Could you check a few things on this drawing? It's one solid part, dimensions in mm from its lowest x, y, z. Round coordinates to 2 decimals unless told otherwise and drop trailing zeros. Loops run counter-clockwise (first coordinate to the right, second up) from the corner with the lowest first, then second, coordinate; pieces in that order, holes last. Notation, with made-up numbers: M 76,9.5 L 95,9.5 A17 cw 95,23.5 Z; hole C 14.5,-3.75 d11. An arc over 180 degrees is marked long. Answer as a JSON object with one key per item and string values.
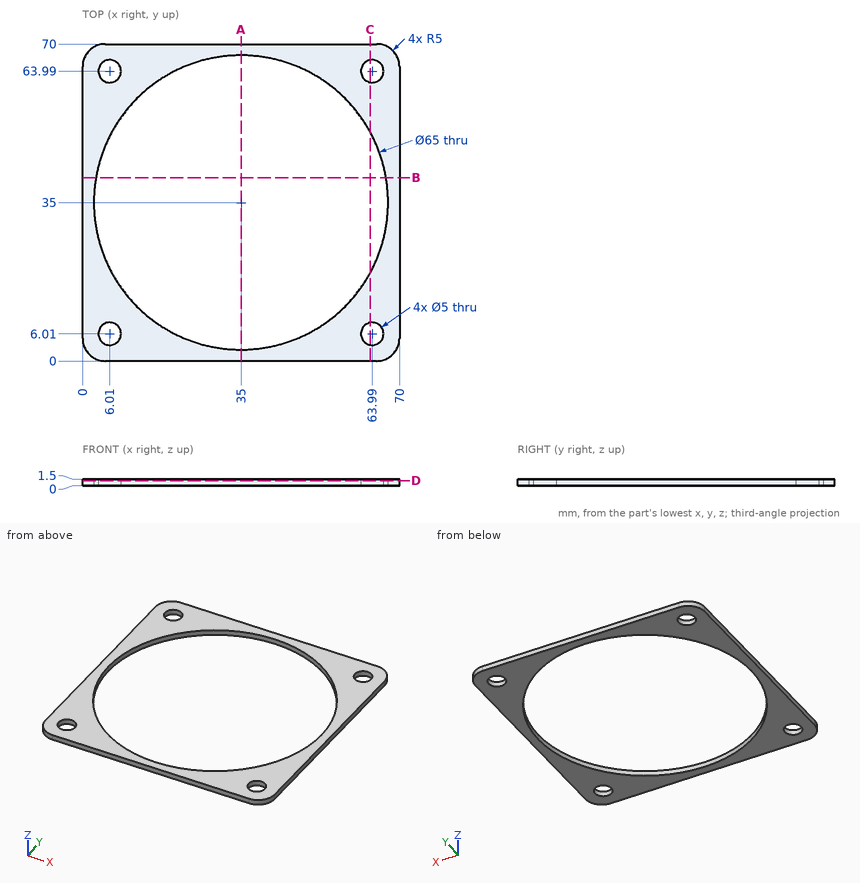
Item 1: I want a section at A-A, the plane x = 35. Please give me the cut outline in (y, z).
Resolved:
{"outline": "M 0,0 L 2.5,0 L 2.5,1.5 L 0,1.5 Z; M 67.5,0 L 70,0 L 70,1.5 L 67.5,1.5 Z"}
Item 2: I want a section at C-C, the plane x = 63.5. Please give me the cut outline in (y, z).
Resolved:
{"outline": "M 0,0 L 3.56,0 L 3.56,1.5 L 0,1.5 Z; M 8.46,0 L 19.38,0 L 19.38,1.5 L 8.46,1.5 Z; M 50.62,0 L 61.54,0 L 61.54,1.5 L 50.62,1.5 Z; M 66.44,0 L 70,0 L 70,1.5 L 66.44,1.5 Z"}
Item 3: I want a section at B-B, the plane y = 40.5. Please give me the cut outline in (x, z).
Resolved:
{"outline": "M 0,0 L 2.97,0 L 2.97,1.5 L 0,1.5 Z; M 67.03,0 L 70,0 L 70,1.5 L 67.03,1.5 Z"}
Item 4: I want a section at D-D, the plane z = 1.15. Please give me the cut outline in (x, y).
Resolved:
{"outline": "M 0,5 A5 ccw 5,0 L 65,0 A5 ccw 70,5 L 70,65 A5 ccw 65,70 L 5,70 A5 ccw 0,65 Z; hole C 35,35 d65; hole C 6.01,6.01 d5; hole C 6.01,63.99 d5; hole C 63.99,6.01 d5; hole C 63.99,63.99 d5"}
Item 5: Please list where these lines run through material, in increasing order: probe 1 along Y at (x, z) = (64, 0.3) (1 decimal); probe 2 along Y at (x, z) = (5, 1.25) (1 decimal); probe 3 along X at (y, z) = (29.5, 0.5). Write a range as from..to.
Resolved:
{"probe 1": "0..3.5, 8.5..20.3, 49.7..61.5, 66.5..70", "probe 2": "0..3.7, 8.3..22.5, 47.5..61.7, 66.3..70", "probe 3": "0..2.97, 67.03..70"}
Item 6: I'm going to push a flat-ended pin straight in: pin 1 Ø6.5 at (x, y) = (63.99, 63.99) entering from -Z. Where does the tip first touch, or does it pass through?
Resolved:
{"pin 1": "z = 0"}
